from build123d import *

# Parameters (mm, degrees)
SKETCH1_W           = 70
SKETCH1_H           = 10
BOSS_EXTRUDE2_DEPTH = 50
SKETCH2_W           = 44
SKETCH2_H           = 44
CUT_EXTRUDE6_DEPTH  = 10
SKETCH3_W           = 44
SKETCH3_H           = 44
CUT_EXTRUDE8_DEPTH  = 12
SKETCH6_W           = 70
SKETCH6_H           = 6
BOSS_EXTRUDE3_DEPTH = 50


with BuildPart() as part:
    # Sketch1 → Boss-Extrude2 (new body)
    with BuildSketch(Plane.XY):
        with BuildLine():
            Line((60.184895573, 46.459182221), (70, 46.459182221))
            Line((70, 46.459182221), (70, 10))
            Line((70, 10), (0, 10))
            Line((0, 10), (0, 46))
            Line((0, 46), (9.701778719, 46))
            ThreePointArc((9.701778719, 46), (35.236479929, 14.00107546), (60.184895573, 46.459182221))
        make_face()
        with Locations((35, 5)):
            Rectangle(SKETCH1_W, SKETCH1_H)
    extrude(amount=BOSS_EXTRUDE2_DEPTH)

    # Sketch2 → Cut-Extrude6 (cut)
    with BuildSketch(Plane(origin=(0, 14, 0), x_dir=(1, 0, 0), z_dir=(0, 1, 0))):
        with Locations((35, -25)):
            Rectangle(SKETCH2_W, SKETCH2_H)
    extrude(amount=CUT_EXTRUDE6_DEPTH, mode=Mode.SUBTRACT)

    # Sketch3 → Cut-Extrude8 (cut)
    with BuildSketch(Plane(origin=(0, 14, 0), x_dir=(1, 0, 0), z_dir=(0, 1, 0))):
        with Locations((35, -25)):
            Rectangle(SKETCH3_W, SKETCH3_H)
    extrude(amount=-CUT_EXTRUDE8_DEPTH, mode=Mode.SUBTRACT)

    # Sketch6 → Boss-Extrude3 (add)
    with BuildSketch(Plane.XY):
        with Locations((35, -3)):
            Rectangle(SKETCH6_W, SKETCH6_H)
    extrude(amount=BOSS_EXTRUDE3_DEPTH)


solid = part.part
Can you work these out from the model? Positions are in its coordinate system, mm. A direction names the side the tool comes from. Round coordinates to 2 decimals unless told otherwise and drop trailing zeros. Loops run counter-clockwise (first coordinate to the right, second up) from the corner with the lowest first, then second, coordinate; pieces in that order, holes last. Notation, with made-up numbers: (41.25, -3) - (55.25, -3) arc R36 ccw to (55.25, 35) - close; hole circle Ø5 at (-5, 12.5). An arc over 180 degrees is marked (long way). Write item = value, one per line. Start each with the question number.
(1) For faces 1 (the face through (13, 13, 25)), 2 (the face through (35, 9, 0)), which set-ups out of +Z, -Z, +X, -X, +Y, -Y let a thin tool reach every point of the face, with its end or its side?
(2) For P1, Ø4, axis at x = 15, z = 31.5, coming from the +Y side; P2, Ø3, axis at x = 5.5, z = 35.5, coming from the +Y side; P3, Ø22, axis at x = 29.5, z = 29, coming from the +Y side, each with a flat end and sliding along its axis, tell me the tip position at first contact or that it passes through.
(3) If I drill on probe 1 along X at (y, z) = (40, 39); probe 2 along Z at (x, y) = (50, 2.5); probe 3 along X at (y, z) = (16, 43), over which ranges is the centre line in solid material (lowest first)? Write a range as [from, to].
(4) If we section it at D-D (y = 34): Please give me the cut outline in (x, z), and give its area (3 significant figures).
(5) If we mould it in two halves opening along Y, with no side actions, what happens to faces 3 (the face through (5, 46, 25)), 4 (the face through (35, 9, 50)), 5 (the face through (57, 13, 25))? For each: released by +Y, released by -Y, zero draft, split by the parting line, or undercut.
(6) If we section it at A-A (y = 40): Please give me the cut outline in (x, z), and give its area (3 significant figures).
(7) If we section it at B-B (z = 36): Please give me the cut outline in (x, y), and give its area (3 significant figures).
(8) If we section it at C-C (x = 19.5): Please give me the cut outline in (y, z), and give its area (3 significant figures).
Ans:
q1.face_1 = none
q1.face_2 = -Z, +X, -X, +Y, -Y
q2.P1 = 26.14
q2.P2 = 46
q2.P3 = 2
q3.probe_1 = [0, 9], [61, 70]
q3.probe_2 = [0, 3], [47, 50]
q3.probe_3 = [0, 13], [57, 70]
q4.outline = (0, 0) - (9.7, 0) - (9.7, 50) - (0, 50) - close; (60.3, 0) - (70, 0) - (70, 50) - (60.3, 50) - close
q4.area = 970 mm²
q5.face_3 = released by +Y
q5.face_4 = zero draft
q5.face_5 = undercut
q6.outline = (0, 0) - (9, 0) - (9, 50) - (0, 50) - close; (61, 0) - (70, 0) - (70, 50) - (61, 50) - close
q6.area = 900 mm²
q7.outline = (0, -6) - (70, -6) - (70, 46.46) - (60.18, 46.46) arc R26 cw to (55.49, 24) - (57, 24) - (57, 2) - (13, 2) - (13, 24) - (14.51, 24) arc R26 cw to (9.7, 46) - (0, 46) - close
q7.area = 1,590 mm²
q8.outline = (-6, 0) - (19.13, 0) - (19.13, 3) - (2, 3) - (2, 47) - (19.13, 47) - (19.13, 50) - (-6, 50) - close
q8.area = 503 mm²
